Work out the finished part from the listing and answer in its coordinate system (mm). Face numbers are marked on the shaded views. A direction names the side the tool comes from. Give positions to 0.01 mm unless a question says otherwise; leave off trailing zeros. Loops run counter-clockwise (first coordinate to the right, second up) from the corner with the lowest first, then second, coordinate; pieces in that order, holes last. Notation, with made-up numbers: M 23,32 L 47,32 A27 ccw 47,49 Z; hole C 75.5,53.5 d2. An arc over 180 degrees is marked long. Answer as a JSON object with one key per item and string values. Group by question number.
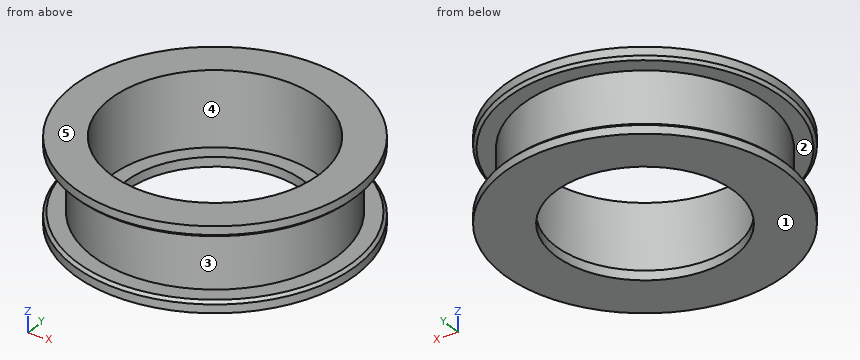
```python
from build123d import *

# Parameters (mm, degrees)
F2_R     = 9.5
F3_DEPTH = 8.9
F2_R_2   = 11.1
F4_DEPTH = 7.9
F5_SIZE  = 0.3


with BuildPart() as f1:
    # F0 (on Front) → F1 (revolve)
    with BuildSketch(Plane.XZ):
        Polygon((15, 4.45), (0, 4.45), (0, -4.45), (15, -4.45), (15, -3.25), (13, -3.25), (13, 3.25), (15, 3.25), align=None)
    revolve(axis=Axis((0, 0, 0), (0, 0, -1)))

    # F2 (on face) → F3 (cut, through all)
    with BuildSketch(Plane.XY.offset(4.45)):
        Circle(F2_R)
    extrude(amount=-F3_DEPTH, mode=Mode.SUBTRACT)

    # F2 (on face) → F4 (cut)
    with BuildSketch(Plane.XY.offset(4.45)):
        Circle(F2_R_2)
        Circle(F2_R, mode=Mode.SUBTRACT)
    extrude(amount=-F4_DEPTH, mode=Mode.SUBTRACT)

    # F5
    f5_edges = [f1.edges().sort_by_distance(p)[0] for p in [
        (-15, 0, -3.25),
        (-15, 0, 3.25),
    ]]
    chamfer(f5_edges, length=F5_SIZE)


solid = f1.part
```
Item 1: A tool of negligible diameter and unlimited length cuts with its end or side. For the marked faces 1 and 2, from which of +Z, -Z, +X, -X, +Y, -Y can it reach the whole face along a straight path? Write none if from no direction.
Item 2: For a pull along Z with two mould halves and no side action, classify the marked faces 3, 4 and 5 as pulls with the +Z half, pulls with the -Z half, needs draft (parallel to the pull), parting line crosses it, or undercut.
Item 3: A cutting plane is placed at C-C (z = -4). Determine the outline of the cut face in (x, y), and give its area (3 significant figures).
Item 4: A cutting plane is placed at A-A (x = 0). Determine the outline of the cut face in (y, z).
Item 5: Given pin 1 Ø13.5 at (x, y) = (0, 0) entering from -Z; pin 2 Ø3 at (x, z) = (4, -2.5) entering from -Y; pin 3 Ø3 at (y, z) = (11.5, 0) entering from -X; pin 4 Ø1.5 at (y, z) = (-2.5, 2) entering from -X, each flat-ended and moving along its own axis, determine where each tip first touches the part or whether it passes through.
Item 6: Find the intervals of material crossed by probe 1 along Z at (x, y) = (13.5, 2.5); probe 2 along Y at (x, z) = (0, 0); probe 3 along Y at (x, z) = (0, -4), in increasing order. Write a range as [from, to].
The answers:
{
 "1": {"face 1": "-Z, +X, -X, +Y, -Y", "face 2": "none"},
 "2": {"face 3": "undercut", "face 4": "needs draft", "face 5": "pulls with the +Z half"},
 "3": {"outline": "C 0,0 d30; hole C 0,0 d19", "area": "423 mm^2"},
 "4": {"outline": "M -15,-4.45 L -9.5,-4.45 L -9.5,-3.45 L -11.1,-3.45 L -11.1,4.45 L -15,4.45 L -15,3.55 L -14.7,3.25 L -13,3.25 L -13,-3.25 L -14.7,-3.25 L -15,-3.55 Z; M 9.5,-4.45 L 15,-4.45 L 15,-3.55 L 14.7,-3.25 L 13,-3.25 L 13,3.25 L 14.7,3.25 L 15,3.55 L 15,4.45 L 11.1,4.45 L 11.1,-3.45 L 9.5,-3.45 Z"},
 "5": {"pin 1": "passes through", "pin 2": "stops at y = -14.71", "pin 3": "stops at x = -8.31", "pin 4": "stops at x = -12.88"},
 "6": {"probe 1": "z = [-4.45, -3.25], [3.25, 4.45]", "probe 2": "y = [-13, -11.1], [11.1, 13]", "probe 3": "y = [-15, -9.5], [9.5, 15]"}
}
